Design review of the part built by this model. Coordinates are the model's own, in mm. Face numbers are marked on the shaded views. A direction names the side the tool comes from. Coordinates: 2 decimals unless noted, no trailing zeros. Order: outer loops, then holes, each group sorted by start corner. A loop starts at its lowest first (then second) coordinate and runs counter-clockwise, first axis right, second up. Notation, with made-up numbers: M 35,55.25 L 71,55.25 A18 cw 71,66.25 Z; hole C 21,43 d7. An arc over 180 degrees is marked long. Answer as a JSON object with one key per item and string values.
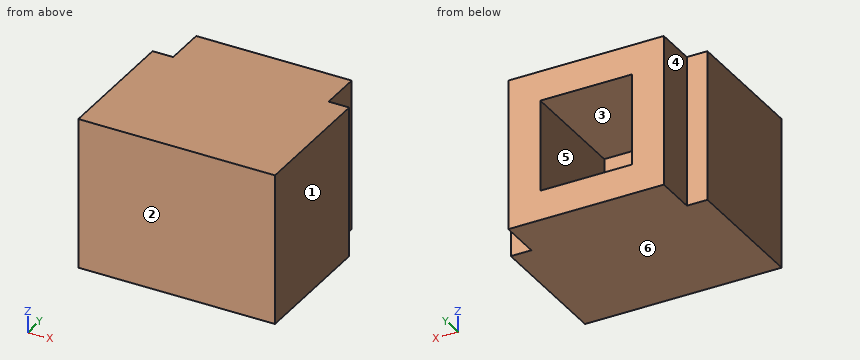
from build123d import *

# Parameters (mm, degrees)
SALIENTE_EXTRUIR1_DEPTH = 66
CROQUIS2_W              = 40
CROQUIS2_H              = 40
CORTAR_EXTRUIR1_DEPTH   = 50


with BuildPart() as part:
    # Croquis1 → Saliente-Extruir1 (new body)
    with BuildSketch(Plane.XY):
        Polygon((-43, -29), (43, -29), (43, 29), (34, 29), (34, 47), (-34, 47), (-34, 29), (-43, 29), align=None)
    extrude(amount=-SALIENTE_EXTRUIR1_DEPTH)

    # Croquis2 → Cortar-Extruir1 (cut)
    with BuildSketch(Plane(origin=(0, 47, 0), x_dir=(1, 0, 0), z_dir=(0, 1, 0))):
        with Locations((0, 33)):
            Rectangle(CROQUIS2_W, CROQUIS2_H)
    extrude(amount=-CORTAR_EXTRUIR1_DEPTH, mode=Mode.SUBTRACT)


solid = part.part
1) To check wall thickness, follow L1, parallel to X at y = 44.5, z = -39.5; L2, parallel to Z at x = 8, y = 34.5; L3, parallel to X at y = 43.5, z = -56. State the ranges of each line that lie inside material, in increasing order.
Taken from the geometry:
{"L1": "x = -34 to -20, 20 to 34", "L2": "z = -66 to -53, -13 to 0", "L3": "x = -34 to 34"}
2) Insertion check: pin 1 Ø2.5 at (x, z) = (37, -30.5) entering from +Y; pin 2 Ø14.5 at (y, z) = (42.5, -40.5) entering from +X; pin 3 Ø14.5 at (y, z) = (37.5, -19.5) entering from -X. Each pin has a flat end and moves straight along its axis. Give the tip position at first contact, or say it passes through.
Taken from the geometry:
{"pin 1": "stops at y = 29", "pin 2": "stops at x = 34", "pin 3": "stops at x = -34"}
3) Add section C-C (x = 6). State the section outline as (y, z) points, and give its area (3 significant figures).
Taken from the geometry:
{"outline": "M -29,-66 L 47,-66 L 47,-53 L -3,-53 L -3,-13 L 47,-13 L 47,0 L -29,0 Z", "area": "3,020 mm2"}
4) Mouldability with a two-part tool opening along X and no side actions: class the marked faces 1, 2 and 3 as released by +X, released by -X, zero draft, split by the parting line, or undercut.
Taken from the geometry:
{"face 1": "released by +X", "face 2": "zero draft", "face 3": "undercut"}
5) Add section B-B (z = -39). State the section outline as (x, y) points.
Taken from the geometry:
{"outline": "M -43,-29 L 43,-29 L 43,29 L 34,29 L 34,47 L 20,47 L 20,-3 L -20,-3 L -20,47 L -34,47 L -34,29 L -43,29 Z"}
6) Add section A-A (y = -1). State the section outline as (x, z) points.
Taken from the geometry:
{"outline": "M -43,-66 L 43,-66 L 43,0 L -43,0 Z; hole M -20,-53 L 20,-53 L 20,-13 L -20,-13 Z"}
7) Tool access review of the marked faces 4, 5 and 6: name each direction out of +Z, -Z, +X, -X, +Y, -Y from which nothing blocks a thin tool from reaching the whole face with its end or side.
Taken from the geometry:
{"face 4": "+Z, -Z, -X, +Y", "face 5": "+Y", "face 6": "-Z, +X, -X, +Y, -Y"}
8) Add section D-D (z = -61.5). State the section outline as (x, y) points, and give its area (3 significant figures).
Taken from the geometry:
{"outline": "M -43,-29 L 43,-29 L 43,29 L 34,29 L 34,47 L -34,47 L -34,29 L -43,29 Z", "area": "6,210 mm2"}
